Can you work these out from the model? Positions are in its coordinate system, mm. Give positions to 0.01 mm unless a question says otherwise; leave off trailing zeros. Loops run counter-clockwise (first coordinate to the right, second up) from the corner with the lowest first, then second, coordinate; pieces in that order, holes last. Notation, with made-up numbers: M 88.25,-3.5 L 137.25,-3.5 A6 ccw 137.25,5.5 Z; hole C 70.25,7 d7. An arc over 180 degrees is marked long. Answer as a JSON object with one key per item and string values.
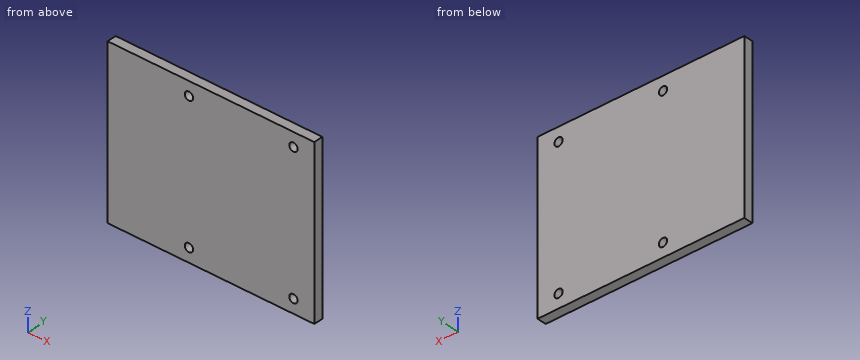
```python
from build123d import *

# Parameters (mm, degrees)
CYLINDER019_R               = 1.8
CYLINDER019_DEPTH           = 20
ARRAY001010_X_COUNT         = 2
ARRAY001010_X_PITCH         = 60
ARRAY001010_Z_COUNT         = 3
ARRAY001010_Z_PITCH         = 45
ARRAY001010_PLACEMENT_ANGLE = 90
BOX011_W                    = 89
BOX011_H                    = 4
BOX011_DEPTH                = 72


with BuildPart() as bottom_hole_array004:
    # Cylinder019 → Cylinder019 (new body)
    with BuildSketch(Plane(origin=(59, 14, 53), x_dir=(1, 0, 0), z_dir=(0, 1, 0))):
        Circle(CYLINDER019_R)
    extrude(amount=CYLINDER019_DEPTH)

    # Array001010 X: bottom hole array004 ×2


with BuildPart() as bottom_hole_array004_1:
    add(bottom_hole_array004.part)
    with Locations(*[(i * ARRAY001010_X_PITCH, 0, 0) for i in range(1, ARRAY001010_X_COUNT)]):
        add(bottom_hole_array004.part)

    # Array001010 Z: bottom hole array004 ×3


with BuildPart() as bottom_hole_array004_2:
    add(bottom_hole_array004_1.part)
    with Locations(*[(0, 0, -i * ARRAY001010_Z_PITCH) for i in range(1, ARRAY001010_Z_COUNT)]):
        add(bottom_hole_array004_1.part)


with BuildPart() as bottom_hole_array004_3:
    # Array001010 placement: moved
    add(bottom_hole_array004_2.part.rotate(Axis((0, 0, 0), (0, 1, 0)), ARRAY001010_PLACEMENT_ANGLE))


with BuildPart() as top_plate_cut002:
    # Box011 → Box011 (new body)
    with BuildSketch(Plane(origin=(-27, 23, -125), x_dir=(1, 0, 0), z_dir=(0, 0, 1))):
        with Locations((44.5, 2)):
            Rectangle(BOX011_W, BOX011_H)
    extrude(amount=BOX011_DEPTH)

    # Cut010: cut bottom hole array004
    add(bottom_hole_array004_3.part, mode=Mode.SUBTRACT)


with BuildPart() as top_plate_cut002_1:
    # Cut010 placement: moved
    add(top_plate_cut002.part.moved(Location((0, 0, 10))))


solid = top_plate_cut002_1.part
```
1) Suppose I cut it at B-B, the plane z = -49. Write out the boundary of the cut face in (x, y).
Answer list:
{"outline": "M -27,23 L 6.2,23 L 6.2,27 L -27,27 Z; M 9.8,23 L 51.2,23 L 51.2,27 L 9.8,27 Z; M 54.8,23 L 62,23 L 62,27 L 54.8,27 Z"}
2) Suppose I cut it at A-A, the plane x = 8. Write out the boundary of the cut face in (y, z), and give its area (3 significant figures).
Answer list:
{"outline": "M 23,-115 L 27,-115 L 27,-110.8 L 23,-110.8 Z; M 23,-107.2 L 27,-107.2 L 27,-50.8 L 23,-50.8 Z; M 23,-47.2 L 27,-47.2 L 27,-43 L 23,-43 Z", "area": "259 mm^2"}
3) Please list where these lines run through material, in increasing order: line 1 along X through (y, z) = (23.9, -109); line 2 along X through (y, z) = (26.65, -107.5). Write a range as from..to.
Answer list:
{"line 1": "-27..6.2, 9.8..51.2, 54.8..62", "line 2": "-27..7.01, 8.99..52.01, 53.99..62"}
4) Will this pin go through, and if not, where does the flat tip stop? pin 1 Ø2 at (x, z) = (53, -49) entering from -Y.
Answer list:
{"pin 1": "through"}
